from build123d import *

# Parameters (mm, degrees)
F0_W     = 12.7
F0_H     = 222.25
F3_W     = 25.4
F3_H     = 3.175
F4_DEPTH = 141.2875
F6_R     = 12.69999
F8_W     = 25.4
F8_H     = 3.175
F9_DEPTH = 141.2875


# Not quite as in the source:
# - a fillet or chamfer is up to 0.001 mm smaller than in the source, because OpenCascade refuses the exact size


with BuildPart() as f1:
    # F0 (on Front) → F1 (revolve)
    with BuildSketch(Plane.XZ):
        with Locations((-6.35, -16.2413566351)):
            Rectangle(F0_W, F0_H)
    revolve(axis=Axis((0, 0, -16.2413566351), (0, 0, -1)))

    # F3 (on Front) → F4 (join, symmetric)
    with BuildSketch(Plane.XZ):
        with Locations((0, 75.8653144777)):
            Rectangle(F3_W, F3_H)
    extrude(amount=F4_DEPTH, both=True)

    # F6 (radius 12.7 in the source; OpenCascade refuses exactly that, so slightly less here)
    f6_edges = [f1.edges().sort_by_distance(p)[0] for p in [
        (12.7, 141.2875, 75.865314),
        (-12.7, 141.2875, 75.865314),
        (-12.7, -141.2875, 75.865314),
        (12.7, -141.2875, 75.865314),
    ]]
    fillet(f6_edges, radius=F6_R)

    # F8 (on line) → F9 (join, symmetric)
    with BuildSketch(Plane(origin=(0, 0, 0), x_dir=(-0.8660254038, 0.5, 0), z_dir=(0.5, 0.8660254038, 0))):
        with Locations((0, 75.8653144777)):
            Rectangle(F8_W, F8_H)
    extrude(amount=F9_DEPTH, both=True)


solid = f1.part
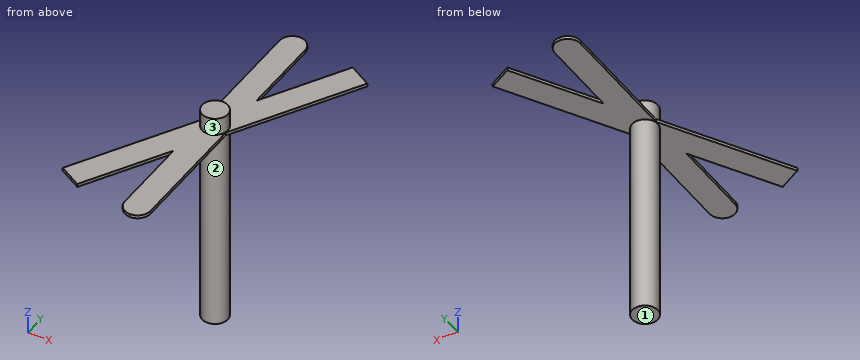
Verification items for the finished model (mm, model axes). Face numbers are marked on the shaded views. A direction names the side the tool comes from. Coordinates: 2 decimals unless noted, no trailing zeros. Order: outer loops, then holes, each group sorted by start corner. A loop starts at its lowest first (then second) coordinate and runs counter-clockwise, first axis right, second up. Notation, with made-up numbers: M 40.5,51.25 L 69.5,51.25 A9 ccw 69.5,56.25 Z; hole C 40.5,11 d11. An arc over 180 degrees is marked long. Return JSON: item names as keys, results as strings.
1) Gauge pin test, flat ends, axial feed: pin 1 (3.5 mm diameter, centred on y = -102.5, z = 75.5, fed in from -X); pin 2 (12 mm diameter, centred on x = 53.5, y = 109.5, fed in from +Z); pin 3 (2.5 mm diameter, centred on y = 87.5, z = 76, fed in from -X). Record the tip position at first contact, or that the pin passes through.
Answer list:
{"pin 1": "x = -74.85", "pin 2": "z = 77.45", "pin 3": "x = -12.7"}
2) Cross-section at C-C, the plane z = -19. Record the boundary of the cut face in (x, y).
Answer list:
{"outline": "C 0,0 d25.4"}
3) Cross-section at B-B, the plane y = 0. Record the boundary of the cut face in (x, z), and give its area (3 significant figures).
Answer list:
{"outline": "M -14.66,74.28 L -12.7,74.28 L -12.7,-127.37 L 12.7,-127.37 L 12.7,74.28 L 14.66,74.28 L 14.66,77.45 L 12.7,77.45 L 12.7,94.88 L -12.7,94.88 L -12.7,77.45 L -14.66,77.45 Z", "area": "5,660 mm2"}
4) Cross-section at A-A, the plane y = -86. Record the boundary of the cut face in (x, z).
Answer list:
{"outline": "M -64.32,74.28 L -34.99,74.28 L -34.99,77.45 L -64.32,77.45 Z; M -12.7,74.28 L 12.7,74.28 L 12.7,77.45 L -12.7,77.45 Z"}
5) Cross-section at D-D, the plane x = -43.5. Record the boundary of the cut face in (y, z).
Answer list:
{"outline": "M -100.74,74.28 L -49.94,74.28 L -49.94,77.45 L -100.74,77.45 Z"}
6) Access from +Z, -Z, +X, -X, +Y, -Y to the whole of each face (thin tool, end or side, straight path). Record for the marked faces 1, 2 and 3.
Answer list:
{"face 1": "-Z, +X, -X, +Y, -Y", "face 2": "-Z", "face 3": "+Z"}
7) Thickness scan on L1, parallel to Z at x = 8.5, y = 109; L2, parallel to X at y = 115.5, z = 75; L3, parallel to X at y = -7.5, z = -81.5. Record the ranges inside material, lowest first. Write a range as [from, to].
Answer list:
{"L1": "[74.28, 77.45]", "L2": "[-12.7, 12.7], [52.02, 81.35]", "L3": "[-10.25, 10.25]"}
